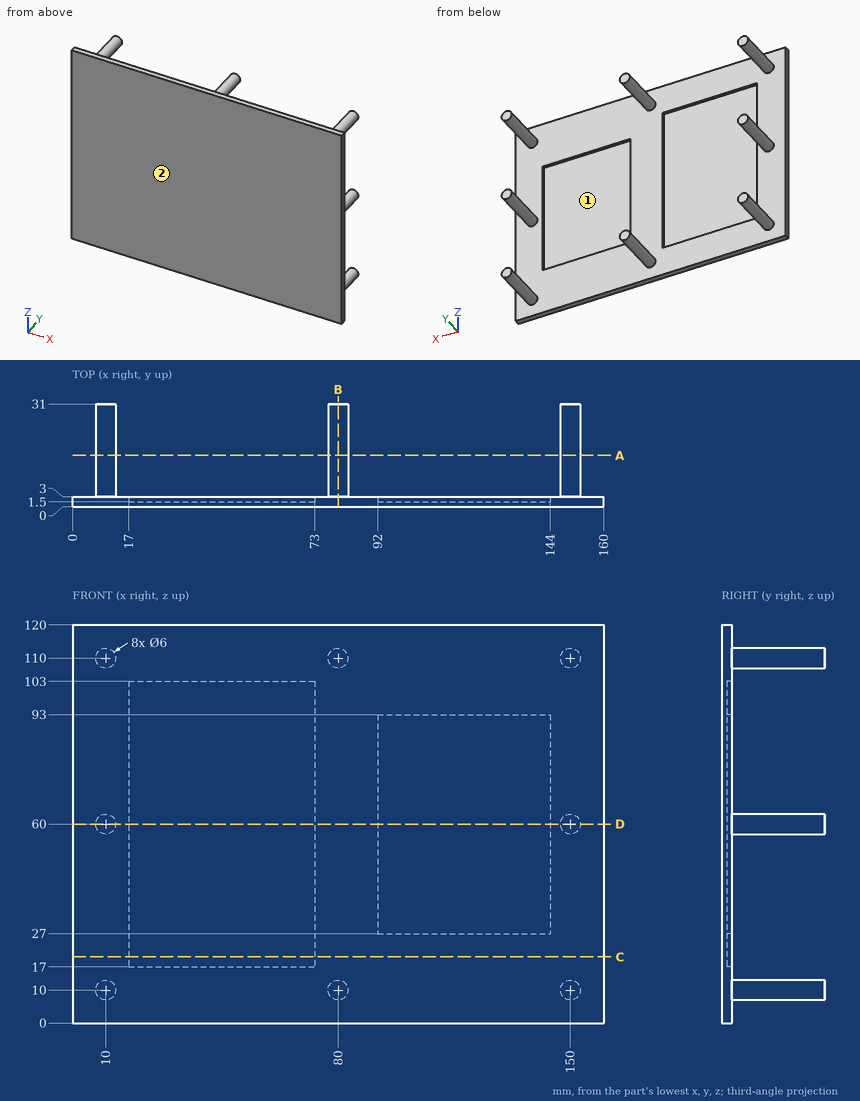
Source: three-view drawing plus pictorial views. Frame: mm from the lowest corner of the part. Round coordinates to 2 decimals unless told otherwise and drop trailing zeros. Loops run counter-clockwise (first coordinate to the right, second up) from the corner with the lowest first, then second, coordinate; pieces in that order, holes last.
Q1. Pin query (flat end, axial travel): P1, Ø12, axis at x = 48, z = 45, coming from the +Y side; P2, Ø6, axis at y = 11.5, z = 56, coming from the +X side; P3, Ø5, axis at x = 83.5, y = 19, coming from the -Z side; P4, Ø10, axis at x = 39, y = 11, coming from the +Z side. Return the tip coordinate at first contact, or that it passes through.
Q2. Pull-direction query (X, two-part tool) for the marked faces 1 and 2; classes: released by +X, released by -X, zero draft, split by the parting line, or undercut.
Q3. Section A-A on y = 15.5. Return loops of the section in (x, z), plus the area to 3 significant figures.
Q4. Section C-C on z = 20. Return loops of the section in (x, y), plus the area to 3 significant figures.
Q5. Section D-D on z = 60. Return loops of the section in (x, y), plus the area to 3 significant figures.
Q6. Section B-B on x = 80. Return loops of the section in (y, z), plus the area to 3 significant figures.
Q7. Material intervals for L1, parallel to X at y = 18.5, z = 108; L2, parallel to Y at x = 18.5, z = 23.5; L3, parallel to X at y = 11, z = 108.5, sorted ascending.
Evaluation:
1. P1: stops at y = 1.5
1. P2: stops at x = 152.83
1. P3: stops at z = 7.17
1. P4: passes through
2. face 1: undercut
2. face 2: zero draft
3. outline: circle Ø6 at (10, 10); circle Ø6 at (10, 60); circle Ø6 at (10, 110); circle Ø6 at (80, 10); circle Ø6 at (80, 110); circle Ø6 at (150, 10); circle Ø6 at (150, 60); circle Ø6 at (150, 110)
3. area: 226 mm2
4. outline: (0, 0) - (160, 0) - (160, 3) - (73, 3) - (73, 1.5) - (17, 1.5) - (17, 3) - (0, 3) - close
4. area: 396 mm2
5. outline: (0, 0) - (160, 0) - (160, 3) - (153, 3) - (153, 31) - (147, 31) - (147, 3) - (144, 3) - (144, 1.5) - (92, 1.5) - (92, 3) - (73, 3) - (73, 1.5) - (17, 1.5) - (17, 3) - (13, 3) - (13, 31) - (7, 31) - (7, 3) - (0, 3) - close
5. area: 654 mm2
6. outline: (0, 0) - (3, 0) - (3, 7) - (31, 7) - (31, 13) - (3, 13) - (3, 107) - (31, 107) - (31, 113) - (3, 113) - (3, 120) - (0, 120) - close
6. area: 696 mm2
7. L1: x = 7.76 to 12.24, 77.76 to 82.24, 147.76 to 152.24
7. L2: y = 0 to 1.5
7. L3: x = 7.4 to 12.6, 77.4 to 82.6, 147.4 to 152.6
